The listing builds one solid part. Answer for the finished solid, in the listing's coordinates (mm). A direction names the side the tool comes from. Coordinates: 2 decimals unless noted, no trailing zeros. Order: outer loops, then holes, each group sorted by start corner. A loop starts at its lowest first (then second) coordinate and runs counter-clockwise, first axis right, second up. Notation, with made-up numbers: M -10.75,80.5 L 3.25,80.5 A29 ccw 3.25,116.5 Z; hole C -2,67 d5. An arc over 180 degrees is marked long. One line per item, written item: value. Start each with the question number.
Q1. The part is cut by section A-A on z = 12.7. Give the vertices of the cut face in (x, y), then the cut area to 3 significant figures.
Q2. Determine the mould class of faces 5 (the flat face through (-32.738, 28.616, 3.444)), 6 (the flat face through (10, 27, 0)), 7 (the flat face through (3, 31, 18.415)), 8 (the flat face through (14, 20.035, 14)) for opening direction Z: pulls with the +Z half, pulls with the -Z half, needs draft (parallel to the pull), parting line crosses it, or undercut.
Q3. The part is cut by section B-B on y = 41.5. Give the number of separate pieces and of enclosed holes in the cut face, then the cut area to 3 significant figures.
Q4. The part is cut by section C-C on x = -24. Give the vertices of the cut face in (y, z) (3 decimals).
Q5. The part is cut by section D-D on z = 21.5. Give the vertices of the cut face in (x, y), then the cut area to 3 significant figures.
Q6. Each of these flat-tipped pins is pushed along its axis until it touches: pin 1 Ø12 at (x, z) = (25.5, 5.5) entering from +Y; pin 2 Ø6.5 at (x, z) = (16.5, 13.5) entering from +Y; pin 3 Ø2.5 at (x, z) = (2.24, 12.7) entering from -Y; pin 4 Ø7.5 at (x, z) = (6.5, 7) entering from -Y. Where does it stop, or does it pass through?
Q7. For faces 1 (the flat face through (38.512, 15, 13)), 2 (the flat face through (0.5, 20.035, 14.4)), 3 (the flat face through (2, 17.005, 10)), 4 (the flat face through (37.183, 1, 13)), determine the directions among +Z, -Z, +X, -X, +Y, -Y from which every point of the face is accessible in a straight line to the end or side of a thin tool.
Q8. Straight lines are drawn through the part: line 1 along X through (y, z) = (19.25, 12.7); line 2 along Z through (x, y) = (15.5, 27.5) (3 decimals); line 3 along X through (y, z) = (11, 13). For each, find the intervals that lie inside material, in ascending order. Write a range as [from, to].
```python
from build123d import *

# Parameters (mm, degrees)
SKETCH1_R                                      = 10.9728
BOSS_EXTRUDE1_DEPTH                            = 25.4
SKETCH2_W                                      = 11.43
SKETCH2_H                                      = 30.40742991
CUT_EXTRUDE1_DEPTH                             = 63.5
CBORE_FOR_8_SOCKET_HEAD_CAP_SCREW2_D           = 4.3053
CBORE_FOR_8_SOCKET_HEAD_CAP_SCREW2_DEPTH       = 7.19576864
CBORE_FOR_8_SOCKET_HEAD_CAP_SCREW2_CBORE_D     = 7.9375
CBORE_FOR_8_SOCKET_HEAD_CAP_SCREW2_CBORE_DEPTH = 4.1656
SKETCH6_W                                      = 7.470933486
SKETCH6_H                                      = 11.420765966
CUT_EXTRUDE2_DEPTH                             = 63.5
SKETCH9_W                                      = 11.43
SKETCH9_H                                      = 7.19576864
CUT_EXTRUDE3_DEPTH                             = 38.1


with BuildPart() as part:
    # Sketch1 → Boss-Extrude1 (new body)
    with BuildSketch(Plane.XY):
        with BuildLine():
            Line((37.182732387, 0.114888998), (37.182732387, 2.802342002))
            Line((37.182732387, 2.802342002), (50.142253344, 34.313558963))
            ThreePointArc((50.142253344, 34.313558963), (39.395041388, 54.329173661), (21.842526976, 39.905698546))
            Line((21.842526976, 39.905698546), (9.430821913, 39.905698546))
            ThreePointArc((9.430821913, 39.905698546), (-5.258087214, 54.594607673), (-19.946996342, 39.905698546))
            Line((-19.946996342, 39.905698546), (-45.891553328, 17.0048778))
            Line((-45.891553328, 17.0048778), (33.346811678, 17.0048778))
            Line((33.346811678, 17.0048778), (33.346811678, 0.114888998))
            Line((33.346811678, 0.114888998), (37.182732387, 0.114888998))
        make_face()
        with BuildLine():
            Line((35.907077172, 25.217162573), (37.182732387, 25.217162573))
            ThreePointArc((37.182732387, 25.217162573), (36.54490478, 25.203320742), (35.907077172, 25.217162573))
        make_face(mode=Mode.SUBTRACT)
        with Locations((-5.258087214, 39.905698546)):
            Circle(SKETCH1_R, mode=Mode.SUBTRACT)
        with Locations((36.54490478, 39.905698546)):
            Circle(SKETCH1_R, mode=Mode.SUBTRACT)
    extrude(amount=BOSS_EXTRUDE1_DEPTH)

    # Sketch2 → Cut-Extrude1 (cut, symmetric)
    with BuildSketch(Plane(origin=(0, 0, 0), x_dir=(0, 0, -1), z_dir=(1, 0, 0))):
        with Locations((-12.7, 39.404361395)):
            Rectangle(SKETCH2_W, SKETCH2_H)
    extrude(amount=CUT_EXTRUDE1_DEPTH, both=True, mode=Mode.SUBTRACT)

    # CBORE for #8 Socket Head Cap Screw2
    with Locations(Plane(origin=(2.23670917, 24.20064644, 12.7), x_dir=(0, 0, 1), z_dir=(0, 1, 0))):
        with Locations((0, 0), (0, 13.971505139)):
            CounterBoreHole(CBORE_FOR_8_SOCKET_HEAD_CAP_SCREW2_D / 2, CBORE_FOR_8_SOCKET_HEAD_CAP_SCREW2_CBORE_D / 2, CBORE_FOR_8_SOCKET_HEAD_CAP_SCREW2_CBORE_DEPTH, depth=CBORE_FOR_8_SOCKET_HEAD_CAP_SCREW2_DEPTH)

    # Sketch6 → Cut-Extrude2 (cut, symmetric)
    with BuildSketch(Plane(origin=(0, 24.20064644, 0), x_dir=(1, 0, 0), z_dir=(0, 1, 0))):
        with Locations((42.247680275, -12.695382983)):
            Rectangle(SKETCH6_W, SKETCH6_H)
    extrude(amount=CUT_EXTRUDE2_DEPTH, both=True, mode=Mode.SUBTRACT)

    # Sketch9 → Cut-Extrude3 (cut)
    with BuildSketch(Plane(origin=(-45.891553328, 0, 0), x_dir=(0, 0, -1), z_dir=(1, 0, 0))):
        with Locations((-12.7, 20.60276212)):
            Rectangle(SKETCH9_W, SKETCH9_H)
    extrude(amount=CUT_EXTRUDE3_DEPTH, mode=Mode.SUBTRACT)


solid = part.part
```
Output:
1. outline: M -7.79,17 L 0.08,17 L 0.08,20.04 L -1.73,20.04 L -1.73,24.2 L -7.79,24.2 Z; M 4.39,17 L 14.06,17 L 14.06,20.04 L 12.24,20.04 L 12.24,24.2 L 6.21,24.2 L 6.21,20.04 L 4.39,20.04 Z; M 18.36,17 L 33.35,17 L 33.35,0.11 L 37.18,0.11 L 37.18,2.8 L 38.51,6.03 L 38.51,24.2 L 20.18,24.2 L 20.18,20.04 L 18.36,20.04 Z
1. area: 322 mm^2
2. face 5: needs draft
2. face 6: pulls with the -Z half
2. face 7: undercut
2. face 8: undercut
3. separate pieces: 8
3. enclosed holes: 0
3. area: 210 mm^2
4. outline: M 17.005,0 L 36.328,0 L 36.328,6.985 L 17.005,6.985 Z; M 17.005,18.415 L 36.328,18.415 L 36.328,25.4 L 17.005,25.4 Z
5. outline: M -45.89,17 L 33.35,17 L 33.35,0.11 L 37.18,0.11 L 37.18,2.8 L 50.14,34.31 A14.7 ccw long 21.84,39.91 L 9.43,39.91 A14.69 ccw -19.95,39.91 Z; hole C -5.26,39.91 d21.95; hole C 36.54,39.91 d21.95; hole M 35.91,25.22 A14.7 ccw 37.18,25.22 Z
5. area: 1,870 mm^2
6. pin 1: stops at y = 53.72
6. pin 2: stops at y = 24.2
6. pin 3: passes through
6. pin 4: stops at y = 17
7. face 1: +X, +Y, -Y
7. face 2: +Y
7. face 3: +Z, -Z, -X, -Y
7. face 4: +Z, -Z, +X, -Y
8. line 1: x = [-7.79, 0.08], [4.39, 14.06], [18.36, 38.51]
8. line 2: z = [0, 6.985], [18.415, 25.4]
8. line 3: x = [33.35, 38.51]
